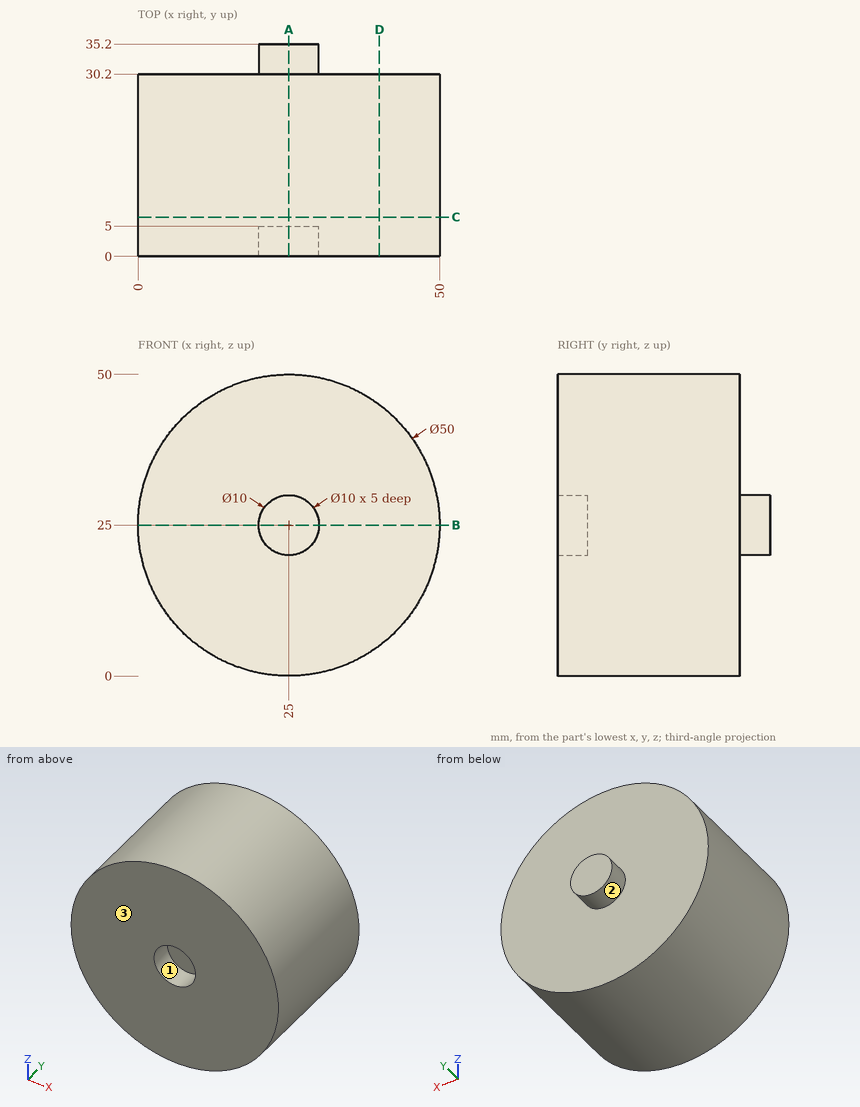
Part print with two shaded views. Sizes in mm from the minimum x, y, z corner. A direction names the side the tool comes from. Give positions to 0.01 mm unless a question says otherwise; leave off trailing zeros. Write each loop counter-clockwise with the first axis right and the second up, starting at its lowest first coordinate (ties: lowest second). Pieces come first, ordered by that corner, then holes.
1) Cut at C-C on y = 6.5. Write the cut outline in (x, z), then the cut area to 3 significant figures.
Resolved:
outline: circle Ø50 at (25, 25)
area: 1,960 mm2
2) Cut at D-D on x = 40. Write the cut outline in (y, z), then the cut area to 3 significant figures.
Resolved:
outline: (0, 5) - (30.2, 5) - (30.2, 45) - (0, 45) - close
area: 1,210 mm2
3) Cut at B-B on z = 25. Write the cut outline in (x, y).
Resolved:
outline: (0, 0) - (20, 0) - (20, 5) - (30, 5) - (30, 0) - (50, 0) - (50, 30.2) - (30, 30.2) - (30, 35.2) - (20, 35.2) - (20, 30.2) - (0, 30.2) - close
4) Which spindle directions (+Z, -Z, +X, -X, +Y, -Y) get a long thin tool onto all of the face, cutting with end or side? Do the marked faces 1, 2 and 3. Say none if no direction does.
Resolved:
face 1: -Y
face 2: +Y
face 3: +Z, -Z, +X, -X, -Y
5) Cut at A-A on x = 25. Write the cut outline in (y, z).
Resolved:
outline: (0, 0) - (30.2, 0) - (30.2, 20) - (35.2, 20) - (35.2, 30) - (30.2, 30) - (30.2, 50) - (0, 50) - (0, 30) - (5, 30) - (5, 20) - (0, 20) - close
6) Probe L1, parallel to Z at x = 25, y = 2; L2, parallel to Y at x = 16, z = 25; L3, parallel to Y at x = 25, z = 24. List the from-to ranges inside material, lowest first.
Resolved:
L1: z = 0 to 20, 30 to 50
L2: y = 0 to 30.2
L3: y = 5 to 35.2
7) Pin check, flat tips, straight feed: pin 1 (1 mm diameter, centred on y = 24, z = 19.5, fed in from +X); pin 2 (4 mm diameter, centred on x = 41, y = 15, fed in from +Z); pin 3 (6 mm diameter, centred on x = 10.5, z = 9.5, fed in from +Y); pin 4 (4 mm diameter, centred on x = 6, z = 23.5, fed in from -Y). Stop position of each tip, or through.
Resolved:
pin 1: stops at x = 49.49
pin 2: stops at z = 45.71
pin 3: stops at y = 30.2
pin 4: stops at y = 0
